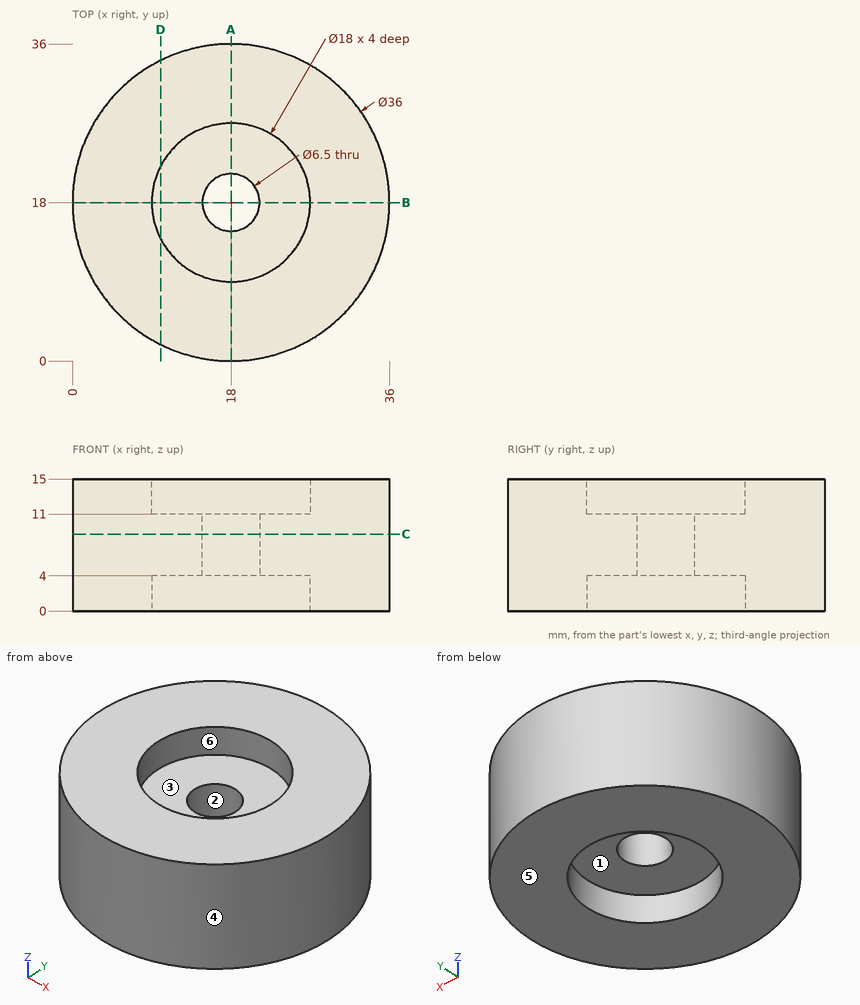
Source: three-view drawing plus pictorial views. Frame: mm from the lowest corner of the part. A direction names the side the tool comes from. Round coordinates to 2 decimals unless told otherwise and drop trailing zeros. Order: outer loops, then holes, each group sorted by start corner. A loop starts at its lowest first (then second) coordinate and runs counter-clockwise, first axis right, second up. Notation, with made-up numbers: (-20, 59) - (-1, 59) arc R18 cw to (-1, 86) - close; hole circle Ø6 at (34, 83). An arc over 180 degrees is marked (long way). Answer in a Markdown table with one row per item.
Item 1: Line query: line 1 (Y direction, x = 18, z = 1.8); line 2 (Z direction, x = 19.5, y = 25); line 3 (X direction, y = 23, z = 3.5). Output: solid intervals per line, ascending.
Model answer:
| item | result |
|---|---|
| line 1 | y = 0 to 9, 27 to 36 |
| line 2 | z = 4 to 11 |
| line 3 | x = 0.71 to 10.52, 25.48 to 35.29 |
Item 2: Mould query, pull axis X, two halves, no side actions, for the marked faces 3, 4, 5 and 6. Classes: released by +X, released by -X, zero draft, split by the parting line, or undercut.
Model answer:
| item | result |
|---|---|
| face 3 | undercut |
| face 4 | split by the parting line |
| face 5 | zero draft |
| face 6 | undercut |
Item 3: Pin query (flat end, axial travel): pin 1 (3 mm diameter, centred on x = 22, y = 22.5, fed in from -Z); pin 2 (5.5 mm diameter, centred on x = 20.5, y = 21.5, fed in from +Z); pin 3 (1 mm diameter, centred on x = 18, z = 7, fed in from -Y). Return the tip coordinate at first contact, or that it passes through.
Model answer:
| item | result |
|---|---|
| pin 1 | stops at z = 4 |
| pin 2 | stops at z = 11 |
| pin 3 | stops at y = 0 |
Item 4: Reachability of the marked faces 1 and 2 from +Z, -Z, +X, -X, +Y, -Y: full face, straight path, thin tool, end or side. Return the list, or none.
Model answer:
| item | result |
|---|---|
| face 1 | -Z |
| face 2 | +Z, -Z |
Item 5: Section query A-A (x = 18). Return the cut outline in (y, z), then the cut area to 4 significant figures.
Model answer:
| item | result |
|---|---|
| outline | (0, 0) - (9, 0) - (9, 4) - (14.75, 4) - (14.75, 11) - (9, 11) - (9, 15) - (0, 15) - close; (21.25, 4) - (27, 4) - (27, 0) - (36, 0) - (36, 15) - (27, 15) - (27, 11) - (21.25, 11) - close |
| area | 350.5 mm² |
Item 6: Section query C-C (z = 8.75). Return the cut outline in (x, y), then the cut area to 3 significant figures.
Model answer:
| item | result |
|---|---|
| outline | circle Ø36 at (18, 18); hole circle Ø6.5 at (18, 18) |
| area | 985 mm² |
Item 7: Section query D-D (x = 10). Return the cut outline in (y, z).
Model answer:
| item | result |
|---|---|
| outline | (1.88, 0) - (13.88, 0) - (13.88, 4) - (22.12, 4) - (22.12, 0) - (34.12, 0) - (34.12, 15) - (22.12, 15) - (22.12, 11) - (13.88, 11) - (13.88, 15) - (1.88, 15) - close |
